from build123d import *

# Parameters (mm, degrees)
SKETCH1_W            = 629.90984
SKETCH1_H            = 147.69846
BOSS_EXTRUDE1_DEPTH  = 3.175
SKETCH3_W            = 254
SKETCH3_H            = 3.175
BOSS_EXTRUDE2_DEPTH  = 6.35
SKETCH4_W            = 3.175
SKETCH4_H            = 188.732840052
CUT_EXTRUDE1_DEPTH   = 3.175
SKETCH6_W            = 3.175
SKETCH6_H            = 110.773845
BOSS_EXTRUDE4_DEPTH  = 3.175
SKETCH8_W            = 629.90984
SKETCH8_H            = 18.04416
BOSS_EXTRUDE5_DEPTH  = 3.175
SKETCH10_W           = 38.1
SKETCH10_H           = 18.04416
SKETCH10_H_2         = 36.08832
CUT_EXTRUDE3_DEPTH   = 652.56536379
BOSS_EXTRUDE6_DEPTH  = 3.175
SKETCH13_R           = 1.55
SKETCH13_R_2         = 11.049
CUT_EXTRUDE4_DEPTH   = 652.56536379
M4_CLEARANCE_HOLE1_D = 4.8


with BuildPart() as part:
    # Sketch1 → Boss-Extrude1 (new body)
    with BuildSketch(Plane(origin=(0, 0, 0), x_dir=(1, 0, 0), z_dir=(0, 1, 0))):
        with Locations((314.95492, 73.84923)):
            Rectangle(SKETCH1_W, SKETCH1_H)
    extrude(amount=BOSS_EXTRUDE1_DEPTH)

    # Sketch3 → Boss-Extrude2 (add)
    with BuildSketch(Plane(origin=(0, 0, -147.69846), x_dir=(-1, 0, 0), z_dir=(0, 0, -1))):
        with Locations((-473.22613, 1.5875)):
            Rectangle(SKETCH3_W, SKETCH3_H)
        with Locations((-156.68371, 1.5875)):
            Rectangle(SKETCH3_W, SKETCH3_H)
    extrude(amount=BOSS_EXTRUDE2_DEPTH)

    # Sketch4 → Cut-Extrude1 (cut)
    with BuildSketch(Plane(origin=(0, 3.175, 0), x_dir=(1, 0, 0), z_dir=(0, 1, 0))):
        with Locations((314.95492, 147.69846)):
            Rectangle(SKETCH4_W, SKETCH4_H)
    extrude(amount=-CUT_EXTRUDE1_DEPTH, mode=Mode.SUBTRACT)

    # Sketch6 → Boss-Extrude4 (add)
    with BuildSketch(Plane(origin=(0, 3.175, 0), x_dir=(1, 0, 0), z_dir=(0, 1, 0))):
        with Locations((631.49734, 92.3115375)):
            Rectangle(SKETCH6_W, SKETCH6_H)
        with Locations((-1.5875, 92.3115375)):
            Rectangle(SKETCH6_W, SKETCH6_H)
    extrude(amount=-BOSS_EXTRUDE4_DEPTH)

    # Sketch8 → Boss-Extrude5 (add, through all)
    with BuildSketch(Plane(origin=(0, 3.175, 0), x_dir=(1, 0, 0), z_dir=(0, 1, 0))):
        with Locations((314.95492, -9.02208)):
            Rectangle(SKETCH8_W, SKETCH8_H)
    extrude(amount=-BOSS_EXTRUDE5_DEPTH)

    # Sketch10 → Cut-Extrude3 (cut, through all)
    with BuildSketch(Plane(origin=(0, 3.175, 0), x_dir=(1, 0, 0), z_dir=(0, 1, 0))):
        with Locations((374.1674, -9.02208)):
            Rectangle(SKETCH10_W, SKETCH10_H)
        with Locations((255.74244, -9.02208)):
            Rectangle(SKETCH10_W, SKETCH10_H)
        with Locations((566.40984, -18.04416)):
            Rectangle(SKETCH10_W, SKETCH10_H_2)
        with Locations((63.5, -18.04416)):
            Rectangle(SKETCH10_W, SKETCH10_H_2)
    extrude(amount=-CUT_EXTRUDE3_DEPTH, mode=Mode.SUBTRACT)

    # Sketch11 → Boss-Extrude6 (add, through all)
    with BuildSketch(Plane(origin=(0, 3.175, 0), x_dir=(1, 0, 0), z_dir=(0, 1, 0))):
        Polygon((0, -18.04416), (0, -137.42416), (629.90984, -137.42416), (629.90984, -18.04416), (585.45984, -18.04416), (585.45984, -27.06624), (547.35984, -27.06624), (547.35984, -18.04416), (393.2174, -18.04416), (393.2174, -27.06624), (355.1174, -27.06624), (355.1174, -18.04416), (274.79244, -18.04416), (274.79244, -26.95194), (236.69244, -26.95194), (236.69244, -18.04416), (82.55, -18.04416), (82.55, -26.95194), (44.45, -26.95194), (44.45, -18.04416), align=None)
    extrude(amount=-BOSS_EXTRUDE6_DEPTH)

    # Sketch13 → Cut-Extrude4 (cut, through all)
    with BuildSketch(Plane.XZ):
        with Locations(Location((227.731580951, 122.331796051, 0), (0, 0, 270))):
            Circle(SKETCH13_R)
        with Locations(Location((250.731580951, 122.331796051, 0), (0, 0, 270))):
            Circle(SKETCH13_R)
        with Locations(Location((227.731580951, 99.331796051, 0), (0, 0, 270))):
            Circle(SKETCH13_R)
        with Locations(Location((250.731580951, 99.331796051, 0), (0, 0, 270))):
            Circle(SKETCH13_R)
        with Locations(Location((152.328523542, 95.877856055, 0), (0, 0, 270))):
            Circle(SKETCH13_R_2)
        with Locations(Location((227.731580951, 79.083184621, 0), (0, 0, 270))):
            Circle(SKETCH13_R)
        with Locations(Location((227.731580951, 56.083184621, 0), (0, 0, 270))):
            Circle(SKETCH13_R)
        with Locations(Location((250.731580951, 56.083184621, 0), (0, 0, 270))):
            Circle(SKETCH13_R)
        with Locations(Location((250.731580951, 79.083184621, 0), (0, 0, 270))):
            Circle(SKETCH13_R)
        with BuildLine():
            Line((245.043121195, 100.323796051), (233.420040708, 100.323796051))
            ThreePointArc((233.420040708, 100.323796051), (227.223580951, 110.831796051), (233.420040708, 121.339796051))
            Line((233.420040708, 121.339796051), (245.043121195, 121.339796051))
            ThreePointArc((245.043121195, 121.339796051), (251.239580951, 110.831796051), (245.043121195, 100.323796051))
        make_face()
        with BuildLine():
            Line((249.739580951, 73.394724865), (249.739580951, 61.771644378))
            ThreePointArc((249.739580951, 61.771644378), (239.231580951, 55.575184621), (228.723580951, 61.771644378))
            Line((228.723580951, 61.771644378), (228.723580951, 73.394724865))
            ThreePointArc((228.723580951, 73.394724865), (239.231580951, 79.591184621), (249.739580951, 73.394724865))
        make_face()
    extrude(amount=-CUT_EXTRUDE4_DEPTH, mode=Mode.SUBTRACT)

    # M4 Clearance Hole1 (through all)
    with Locations(Plane(origin=(0, 0, 0), x_dir=(-1, 0, 0), z_dir=(0, -1, 0))):
        with Locations((-618.09884, -38.11016), (-466.52688, -38.11016), (-618.09884, -127.26416), (-466.52688, -127.26416), (-314.95492, -127.26416), (-314.95492, -38.11016), (-163.38296, -38.11016), (-11.811, -38.11016), (-11.811, -127.26416), (-163.38296, -127.26416)):
            Hole(M4_CLEARANCE_HOLE1_D / 2)


solid = part.part
Verification items for the finished model (mm, model axes). Round coordinates to 2 decimals unless told otherwise and drop trailing zeros. Loops run counter-clockwise (first coordinate to the right, second up) from the corner with the lowest first, then second, coordinate; pieces in that order, holes last. Notation, with made-up numbers: (-26.75, -6.5) - (-2.75, -6.5) arc R23 ccw to (-2.75, 23.5) - close; hole circle Ø4 at (-27, 7.5). An arc over 180 degrees is marked (long way). Answer in a Markdown table with one row per item. Add a question column.
Q1. Material ranges on line 1 (X direction, y = 1.8, z = 37.5); line 2 (X direction, y = 0.4, z = 69.5); line 3 (X direction, y = 2.6, z = -113.5) (3 decimals), recorded low to high.
Q2. Section check B-B on x = 371.5. Enter the section's corners in (y, z) (3 decimals).
Q3. Release check for a two-part mould opening along X. For faces 1 (the face through (311, 0, -10)), 2 (the face through (163.284, 1.565, 97.316)) record: pulls with the +X half, pulls with the -X half, needs draft (parallel to the pull), parting line crosses it, or undercut.
Q4. Section check A-A on z = 17.5. Enter the section's corners in (x, y) (3 decimals), plus the area to 3 significant figures.
Q5. Gauge pin test, flat ends, axial feed: pin 1 (1 mm diameter, centred on x = 337.5, y = 1.5, fed in from -Z); pin 2 (1.5 mm diameter, centred on y = 1, z = 42.5, fed in from +X); pin 3 (3 mm diameter, centred on x = 227.73, z = 79.08, fed in from +Y); pin 4 (1 mm diameter, centred on y = 2, z = -152, fed in from -X). Record the tip position at first contact, or that the pin passes through.
Q6. Section check C-C on x = 301.5. Enter the section's corners in (y, z) (3 decimals), plus the area to 3 significant figures.
Q7. Section check D-D on y = 0.7. State how many separate pieces and enclosed holes the cut face has, plus the area to 3 significant figures.
Found:
| question | item | result |
|---|---|---|
| 1 | line 1 | x = 0 to 9.49, 14.13 to 161.06, 165.7 to 312.63, 317.28 to 464.21, 468.85 to 615.78, 620.42 to 629.91 |
| 1 | line 2 | x = 0 to 228.72, 249.74 to 629.91 |
| 1 | line 3 | x = -3.175 to 313.367, 316.542 to 633.085 |
| 2 | outline | (0, -154.048) - (3.175, -154.048) - (3.175, 0) - (0, 0) - close; (0, 27.066) - (3.175, 27.066) - (3.175, 137.424) - (0, 137.424) - close |
| 3 | face 1 | needs draft |
| 3 | face 2 | undercut |
| 4 | outline | (0, 0) - (44.45, 0) - (44.45, 3.175) - (0, 3.175) - close; (82.55, 0) - (236.692, 0) - (236.692, 3.175) - (82.55, 3.175) - close; (274.792, 0) - (355.117, 0) - (355.117, 3.175) - (274.792, 3.175) - close; (393.217, 0) - (547.36, 0) - (547.36, 3.175) - (393.217, 3.175) - close; (585.46, 0) - (629.91, 0) - (629.91, 3.175) - (585.46, 3.175) - close |
| 4 | area | 1,520 mm² |
| 5 | pin 1 | stops at z = -147.7 |
| 5 | pin 2 | stops at x = 629.91 |
| 5 | pin 3 | passes through |
| 5 | pin 4 | stops at x = 29.68 |
| 6 | outline | (0, -147.698) - (3.175, -147.698) - (3.175, 137.424) - (0, 137.424) - close |
| 6 | area | 905 mm² |
| 7 | separate pieces | 1 |
| 7 | enclosed holes | 25 |
| 7 | area | 178,000 mm² |
